from build123d import *

# Parameters (mm, degrees)
BOSS_EXTRUDE1_DEPTH  = 3.175
M3_CLEARANCE_HOLE1_D = 3.4


with BuildPart() as part:
    # Sketch2 → Boss-Extrude1 (new body)
    with BuildSketch(Plane(origin=(0, 0, 0), x_dir=(1, 0, 0), z_dir=(0, 1, 0))):
        with BuildLine():
            Line((0, 0), (0, 177.8))
            Line((0, 177.8), (-177.8, 177.8))
            ThreePointArc((-177.8, 177.8), (-266.7, 88.9), (-177.8, 0))
            Line((-177.8, 0), (0, 0))
        make_face()
    extrude(amount=BOSS_EXTRUDE1_DEPTH)

    # M3 Clearance Hole1 (through all)
    with Locations(Plane(origin=(0, 3.175, 0), x_dir=(1, 0, 0), z_dir=(0, 1, 0))):
        with Locations((-63.5, 154.95524), (-19.05, 154.95524), (-56.515, 133.36524), (-26.035, 133.36524), (-56.515, 44.43476), (-26.035, 44.43476), (-63.5, 22.84476), (-19.05, 22.84476), (-234.95, 108.9), (-234.95, 68.9)):
            Hole(M3_CLEARANCE_HOLE1_D / 2)


solid = part.part
Geometry check sheet. Reference: the model listing, model coordinates, mm. Round coordinates to 2 decimals unless told otherwise and drop trailing zeros. Order: outer loops, then holes, each group sorted by start corner. A loop starts at its lowest first (then second) coordinate and runs counter-clockwise, first axis right, second up. Notation, with made-up numbers: M 65,-15 L 77,-15 A10 ccw 77,1 Z; hole C 44.5,-15 d8. An arc over 180 degrees is marked long. Answer in a Markdown table with one row per item. Add a question column.
Item 1: Sectioned sample at C-C, the plane z = -147.5. Enter the section's corners in (x, y) (3 decimals).
Item 2: Sectioned sample at B-B, the plane x = -206.5. Enter the section's corners in (y, z) (3 decimals), plus the area to 3 significant figures.
Item 3: Sectioned sample at A-A, the plane y = 1.95. State how many separate pieces and enclosed holes the cut face has, plus the area to 3 significant figures.
Item 4: Material ranges on L1, parallel to Z at x = -234.95, y = 2.3; L2, parallel to Z at x = -57, y = 2.35; L3, parallel to X at y = 2.8, z = -22, recorded low to high. Write a range as [from, to].
Filled in:
| question | item | result |
|---|---|---|
| 1 | outline | M -244.652,0 L 0,0 L 0,3.175 L -244.652,3.175 Z |
| 2 | outline | M 0,-173.04 L 3.175,-173.04 L 3.175,-4.76 L 0,-4.76 Z |
| 2 | area | 534 mm² |
| 3 | separate pieces | 1 |
| 3 | enclosed holes | 10 |
| 3 | area | 43,900 mm² |
| 4 | L1 | z = [-157, -110.6], [-107.2, -70.6], [-67.2, -20.8] |
| 4 | L2 | z = [-177.8, -134.99], [-131.74, -46.06], [-42.81, 0] |
| 4 | L3 | x = [-236.35, -64.98], [-62.02, -20.53], [-17.57, 0] |
